from build123d import *

# Parameters (mm, degrees)
SKETCH1_R            = 210
SKETCH1_R_2          = 190
BOSS_EXTRUDE1_DEPTH  = 5
M6_CLEARANCE_HOLE1_D = 6.6
CUT_EXTRUDE1_DEPTH   = 5
CIRPATTERN1_COUNT    = 8


with BuildPart() as part:
    # Sketch1 → Boss-Extrude1 (new body)
    with BuildSketch(Plane.XY):
        Circle(SKETCH1_R)
        Circle(SKETCH1_R_2, mode=Mode.SUBTRACT)
    extrude(amount=BOSS_EXTRUDE1_DEPTH)

    # M6 Clearance Hole1 (through all)
    with Locations(Plane.XY.offset(5)):
        with Locations((0, 200)):
            m6_clearance_hole1 = Hole(M6_CLEARANCE_HOLE1_D / 2)

    # Sketch4 → Cut-Extrude1 (cut)
    with BuildSketch(Plane.XY.offset(5)):
        with BuildLine():
            ThreePointArc((5.165561681, 196.632161592), (15.742672541, 199.530216011), (5.41785296, 203.227795514))
            ThreePointArc((5.41785296, 203.227795514), (2.709167039, 203.281948077), (0, 203.3))
            ThreePointArc((0, 203.3), (3.3, 200), (0, 196.7))
            ThreePointArc((0, 196.7), (2.583003558, 196.683039667), (5.165561681, 196.632161592))
        make_face()
    cut_extrude1 = extrude(amount=-CUT_EXTRUDE1_DEPTH, mode=Mode.SUBTRACT)

    # CirPattern1: M6 Clearance Hole1, Cut-Extrude1 ×8 about axis
    cirpattern1_axis = Axis((0, 0, 0), (0, 0, 1))
    for i in range(1, CIRPATTERN1_COUNT):
        add(m6_clearance_hole1.rotate(cirpattern1_axis, i * 360 / CIRPATTERN1_COUNT), mode=Mode.SUBTRACT)
        add(cut_extrude1.rotate(cirpattern1_axis, i * 360 / CIRPATTERN1_COUNT), mode=Mode.SUBTRACT)


solid = part.part
Build history of the part. All positions in model axes, mm. Coordinates: 2 decimals unless noted, no trailing zeros. Write each loop counter-clockwise with the first axis right and the second up, starting at its lowest first coordinate (ties: lowest second). Pieces come first, ordered by that corner, then holes.
(1) Cut at C-C on z = 4.1. State how many separate pieces and enclosed holes the cut face has, and give its area (3 significant figures).
(2) Pin check, flat tips, straight feed: pin 1 Ø2 at (x, z) = (-34, 1) entering from +Y; pin 2 Ø1 at (x, z) = (84, 4.5) entering from -Y; pin 3 Ø13 at (x, y) = (-199.75, 10) entering from -Z. Stop position of each tip, or through.
(3) Cut at A-A on x = -51. List the corners of the cut face in (y, z).
(4) Mould opens along X. For faces 1 (the cylindrical face through (129.82, -152.07, 2.54)), 2 (the flat face through (-188, -30, 5)), 3 (the cylindrical face through (200.3, 63.08, 2.46)) say: pulls with the +X half, pulls with the -X half, needs draft (parallel to the pull), parting line crosses it, or undercut.
(5) Drill centre lines: line 1 (X direction, y = 3.5, z = 3.95); line 2 (Y direction, x = 143, z = 4.05); line 3 (Y direction, x = 8.5, z = 4.25). Where is each one in solid material? Low to high.
(6) Cut at B-B on y = -122. List the corners of the cut face in (x, z), and give its area (3 significant figures).
Working result:
1. separate pieces: 1
1. enclosed holes: 9
1. area: 23,900 mm2
2. pin 1: stops at y = 207.39
2. pin 2: stops at y = -192.69
2. pin 3: stops at z = 0
3. outline: (-203.71, 0) - (-183.03, 0) - (-183.03, 5) - (-203.71, 5) - close; (183.03, 0) - (203.71, 0) - (203.71, 5) - (183.03, 5) - close
4. face 1: undercut
4. face 2: needs draft
4. face 3: parting line crosses it
5. line 1: x = -209.97 to -203.27, -196.67 to -189.97, 189.97 to 209.97
5. line 2: y = -153.79 to -144.51, -138.52 to -125.1, 125.1 to 131.98, 144.32 to 153.79
5. line 3: y = -209.83 to -189.81, 189.81 to 194.2, 205.3 to 209.83
6. outline: (-170.93, 0) - (-145.66, 0) - (-145.66, 5) - (-170.93, 5) - close; (145.66, 0) - (170.93, 0) - (170.93, 5) - (145.66, 5) - close
6. area: 253 mm2
